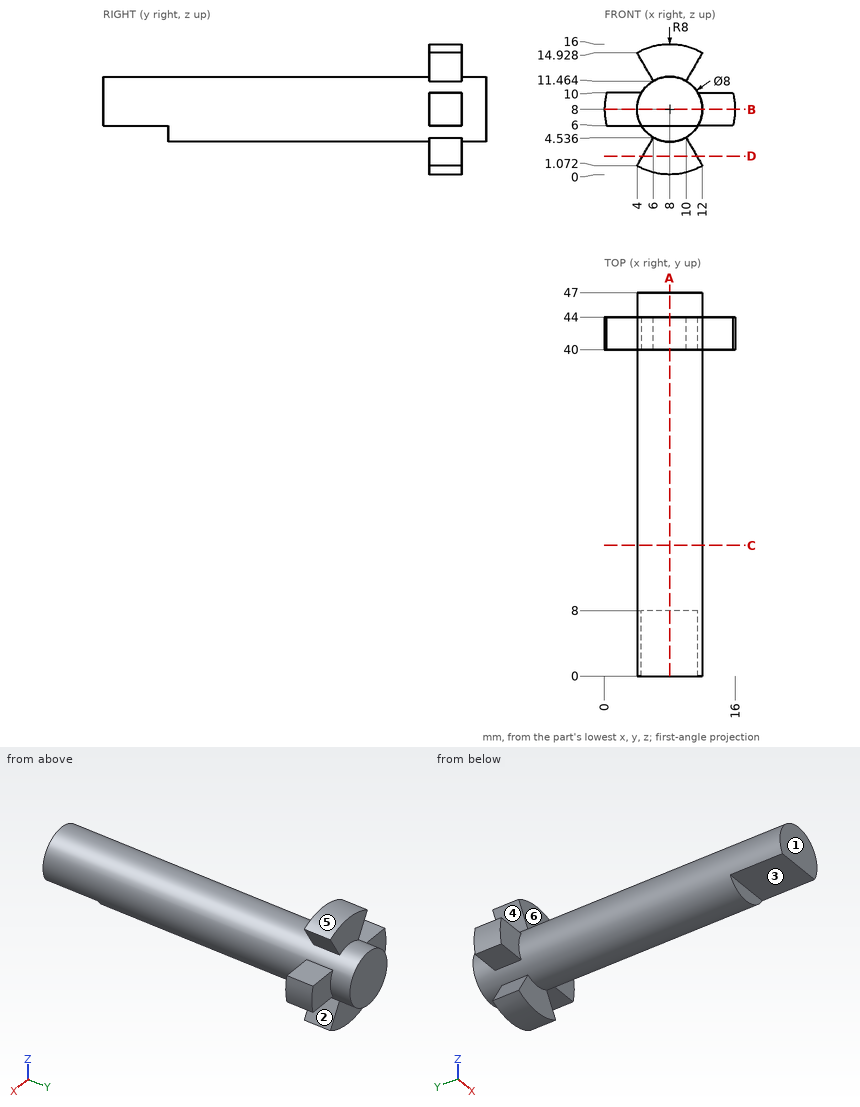
Here's the drawing with two shaded views (mm, measured from the low corner). I have some questions. A direction names the side the tool comes from. Give positions to 0.01 mm unless a question says otherwise; leave off trailing zeros. Loops run counter-clockwise (first coordinate to the right, second up) from the corner with the lowest first, then second, coordinate; pieces in that order, holes last. Notation, with made-up numbers: M 78,9 L 126,9 A10 cw 126,17 Z; hole C -9,-21 d10. An arc over 180 degrees is marked long. Use one line per item in the form item = value. Start each with the question number.
(1) I want a section at A-A, the plane x = 8. Write out the boundary of the cut face in (y, z).
(2) I want a section at C-C, the plane y = 16. Write out the boundary of the cut face in (x, z).
(3) Please list where these lines run through material, in increasing order: line 1 (Y direction, x = 13.5, z = 6.25); line 2 (Y direction, x = 10.5, z = 5.25); line 3 (X direction, y = 13, z = 7.75).
(4) I want a section at B-B, the plane z = 8. Write out the boundary of the cut face in (x, y).
(5) Thinking about a two-plate mould opening in Z: for the marked faces 3, 4, 5 and 6, which applies, released by +Z, released by -Z, zero draft, split by the parting line, or undercut?
(6) I want a section at D-D, the plane z = 2.25. Write out the boundary of the cut face in (x, y).
(7) On a 3-axis mill with a long thin cutter (end or side, diameter ignored), from which of +Z, -Z, +X, -X, +Y, -Y can I reach the whole of each face in a straight line? I mean the marked faces 1 and 2. Say none if no direction works.
(8) I'm going to push flat-ended pins straight in: P1, Ø2, axis at x = 2, z = 7.5, coming from the -Y side; P2, Ø4.5, axis at x = 1.5, y = 41.5, coming from the -Z side; P3, Ø6, axis at y = 11.5, z = 10.5, coming from the +X side. Where does each tip first touch, or does it pass through?
Worked out:
q1.outline = M 0,6 L 8,6 L 8,4 L 40,4 L 40,0 L 44,0 L 44,4 L 47,4 L 47,12 L 44,12 L 44,16 L 40,16 L 40,12 L 0,12 Z
q2.outline = C 8,8 d8
q3.line_1 = 40 to 44
q3.line_2 = 8 to 47
q3.line_3 = 4.01 to 11.99
q4.outline = M 0,40 L 4,40 L 4,0 L 12,0 L 12,40 L 16,40 L 16,44 L 12,44 L 12,47 L 4,47 L 4,44 L 0,44 Z
q5.face_3 = released by -Z
q5.face_4 = undercut
q5.face_5 = released by +Z
q5.face_6 = zero draft
q6.outline = M 4.68,40 L 11.32,40 L 11.32,44 L 4.68,44 Z
q7.face_1 = +Z, -Z, +X, -X, -Y
q7.face_2 = +X, +Y, -Y
q8.P1 = 40
q8.P2 = 6
q8.P3 = 12
